Read the model definition and answer for the solid it produces. Units are mm, in the model's axes. A direction names the side the tool comes from. Round coordinates to 2 decimals unless told otherwise and drop trailing zeros. Write each loop counter-clockwise with the first axis right and the second up, starting at its lowest first coordinate (ties: lowest second). Pieces come first, ordered by that corner, then holes.
from build123d import *

# Parameters (mm, degrees)
SKETCH005_R   = 100
SKETCH005_R_2 = 10
PAD003_DEPTH  = 200
SKETCH010_R   = 150
SKETCH010_R_2 = 10
PAD007_DEPTH  = 1
SKETCH011_R   = 150
PAD008_DEPTH  = 1


with BuildPart() as part:
    # Sketch005 → Pad003 (new body)
    with BuildSketch(Plane.YZ):
        Circle(SKETCH005_R)
        Circle(SKETCH005_R_2, mode=Mode.SUBTRACT)
    extrude(amount=PAD003_DEPTH)

    # Sketch010 (on Face3 of Pad003) → Pad007 (join)
    with BuildSketch(Plane(origin=(0, 0, 0), x_dir=(0, 1, 0), z_dir=(-1, 0, 0))):
        Circle(SKETCH010_R)
        Circle(SKETCH010_R_2, mode=Mode.SUBTRACT)
    extrude(amount=PAD007_DEPTH)

    # Sketch011 (on Face3 of Pad007) → Pad008 (join)
    with BuildSketch(Plane.YZ.offset(200)):
        Circle(SKETCH011_R)
    extrude(amount=PAD008_DEPTH)


with BuildPart() as part_1:
    # Body002 placement: moved
    add(part.part.moved(Location((0, -225, 160))))


solid = part_1.part
Q1. Flat-ended cylindrical pins translate along their axes: pin 1 Ø2 at (x, z) = (158.5, 113) entering from -Y; pin 2 Ø5 at (x, z) = (80.5, 141.5) entering from +Y; pin 3 Ø4 at (x, z) = (54, 98) entering from +Y. Find the tip coordinate at first contact, or state that the pin passes through.
Verdict:
pin 1: stops at y = -313.79
pin 2: stops at y = -126.29
pin 3: stops at y = -145
Q2. Section C-C (y = -225) is taken. Determine the outline of the cut face in (x, z).
Verdict:
outline: (-1, 10) - (0, 10) - (0, 60) - (200, 60) - (200, 10) - (201, 10) - (201, 310) - (200, 310) - (200, 260) - (0, 260) - (0, 310) - (-1, 310) - (-1, 170) - (200, 170) - (200, 150) - (-1, 150) - close
Q3. Determine the mould class of faces 1 (the cylindrical face through (200.493, -86.438, 102.549)), 2 (the cylindrical face through (100.907, -215.763, 163.83)), 3 (the flat face through (-1, -194, 158)) for opening direction Y: pulls with the +Y half, pulls with the -Y half, needs draft (parallel to the pull), parting line crosses it, or undercut.
Verdict:
face 1: parting line crosses it
face 2: undercut
face 3: needs draft
Q4. Section A-A (z = 289) is taken. Determine the outline of the cut face in (x, y), then the cut area to 3 significant figures.
Verdict:
outline: (-1, -301.54) - (0, -301.54) - (0, -148.46) - (-1, -148.46) - close; (200, -301.54) - (201, -301.54) - (201, -148.46) - (200, -148.46) - close
area: 306 mm2
Q5. Section D-D (z = 160) is taken. Determine the outline of the cut face in (x, y), then the cut area to 3 significant figures.
Verdict:
outline: (-1, -375) - (0, -375) - (0, -325) - (200, -325) - (200, -375) - (201, -375) - (201, -75) - (200, -75) - (200, -125) - (0, -125) - (0, -75) - (-1, -75) - (-1, -215) - (200, -215) - (200, -235) - (-1, -235) - close
area: 36,600 mm2
Q6. Section B-B (x = 134) is taken. Determine the outline of the cut face in (y, z).
Verdict:
outline: circle Ø200 at (-225, 160); hole circle Ø20 at (-225, 160)
Q7. Straight lines are drawn through the part: probe 1 along X at (y, z) = (-324.5, 127); probe 2 along Z at (x, y) = (150, -225); probe 3 along Y at (x, z) = (88, 164). For each, find the intervals that lie inside material, in ascending order.
Verdict:
probe 1: x = -1 to 0, 200 to 201
probe 2: z = 60 to 150, 170 to 260
probe 3: y = -324.92 to -234.17, -215.83 to -125.08
Q8. Which of the six approach directions +Z, -Z, +X, -X, +Y, -Y give full straight-line access (tool end or side, diameter ignored) to faces 4 (the flat face through (201, -227, 162)), 5 (the cylindrical face through (98.6, -304.357, 99.152)), 6 (the flat face through (200, -225, 160))?
Verdict:
face 4: +Z, -Z, +X, +Y, -Y
face 5: none
face 6: -X
